```python
from build123d import *

# Parameters (mm, degrees)
SKETCH1_R           = 2
BOSS_EXTRUDE1_DEPTH = 2.5


with BuildPart() as part:
    # Sketch1 → Boss-Extrude1 (new body)
    with BuildSketch(Plane(origin=(0, 0, 0), x_dir=(1, 0, 0), z_dir=(0, 1, 0))):
        with BuildLine():
            Line((-2, -4.582575695), (-2, -36))
            Line((-2, -36), (-4, -36))
            Line((-4, -36), (-4, -42))
            Line((-4, -42), (4, -42))
            Line((4, -42), (4, -36))
            Line((4, -36), (2, -36))
            Line((2, -36), (2, -4.582575695))
            ThreePointArc((2, -4.582575695), (4.83465237, -1.275200556), (4, 3))
            Line((4, 3), (4, 30))
            Line((4, 30), (5.25505198, 32.173813795))
            Line((5.25505198, 32.173813795), (3.75505198, 33.039839198))
            Line((3.75505198, 33.039839198), (2, 30))
            Line((2, 30), (-2, 30))
            Line((-2, 30), (-3.75505198, 33.039839198))
            Line((-3.75505198, 33.039839198), (-5.25505198, 32.173813795))
            Line((-5.25505198, 32.173813795), (-4, 30))
            Line((-4, 30), (-4, 3))
            ThreePointArc((-4, 3), (-4.83465237, -1.275200556), (-2, -4.582575695))
        make_face()
        with Locations(Location((0, 0, 0), (0, 0, 270))):
            Circle(SKETCH1_R, mode=Mode.SUBTRACT)
    extrude(amount=BOSS_EXTRUDE1_DEPTH)


solid = part.part
```
Source: CAD feature listing. Evaluate the final solid. Frame: model axes, mm. A direction names the side the tool comes from. Round coordinates to 2 decimals unless told otherwise and drop trailing zeros. Loops run counter-clockwise (first coordinate to the right, second up) from the corner with the lowest first, then second, coordinate; pieces in that order, holes last.
(1) Section query B-B (y = 0.45). Output: boundary loops of the cut face in (x, z).
From the geometry:
outline: (-5.26, -32.17) - (-3.76, -33.04) - (-2, -30) - (2, -30) - (3.76, -33.04) - (5.26, -32.17) - (4, -30) - (4, -3) arc R5 ccw to (2, 4.58) - (2, 36) - (4, 36) - (4, 42) - (-4, 42) - (-4, 36) - (-2, 36) - (-2, 4.58) arc R5 ccw to (-4, -3) - (-4, -30) - close; hole circle Ø4 at (0, 0)
(2) Section query C-C (z = 0). Output: boundary loops of the cut face in (x, y).
From the geometry:
outline: (-5, 0) - (-2, 0) - (-2, 2.5) - (-5, 2.5) - close; (2, 0) - (5, 0) - (5, 2.5) - (2, 2.5) - close
(3) Access query for faces 1 (the flat face through (4, 1, -16)), 2 (the flat face through (4, 1, 39)), 3 (the flat face through (-2.865, 1.232, -31.499)), 4 (the flat face through (-4, 1, -17)). Directions: +Z, -Z, +X, -X, +Y, -Y. A direction counts if a zero-diameter tool reaches every point of the face in a straight line with its end or side. Return the directions, or none.
From the geometry:
face 1: +X, +Y, -Y
face 2: +Z, +X, +Y, -Y
face 3: -Z, +Y, -Y
face 4: -X, +Y, -Y
(4) Pull-direction query (Z, two-part tool) for faces 5 (the flat face through (-4, 1, 39)), 6 (the flat face through (0, 1, 42)), 7 (the flat face through (0, 1, -30)), 8 (the cylindrical face through (-4.85, 1.23, 1.21)); classes: +Z half, -Z half, draft (parallel to the pull), parting line (faces both ways), or undercut.
From the geometry:
face 5: draft
face 6: +Z half
face 7: -Z half
face 8: undercut
(5) Section query A-A (x = 0). Output: boundary loops of the cut face in (y, z), and give its area (3 significant figures).
From the geometry:
outline: (0, -30) - (2.5, -30) - (2.5, -2) - (0, -2) - close; (0, 2) - (2.5, 2) - (2.5, 42) - (0, 42) - close
area: 170 mm2
(6) Section query D-D (z = -12). Output: boundary loops of the cut face in (x, y).
From the geometry:
outline: (-4, 0) - (4, 0) - (4, 2.5) - (-4, 2.5) - close
(7) Contact query for flat-ended pins moving along their axis: pin 1 Ø0.8 at (y, z) = (1, -11) entering from +X; pin 2 Ø1.2 at (y, z) = (1, 40) entering from -X; pin 3 Ø1.2 at (x, y) = (0.5, 1.5) entering from -Z. Output: stop coordinate, or through.
From the geometry:
pin 1: stops at x = 4
pin 2: stops at x = -4
pin 3: stops at z = -30
(8) Material intervals for probe 1 along X at (y, z) = (1.75, 0); probe 2 along Z at (x, y) = (-0.25, 2.05); probe 3 along X at (y, z) = (0.4, -24.5), sorted ascending.
From the geometry:
probe 1: x = -5 to -2, 2 to 5
probe 2: z = -30 to -1.98, 1.98 to 42
probe 3: x = -4 to 4
